```python
from build123d import *

# Parameters (mm, degrees)
F0_W     = 165
F0_H     = 100
F1_DEPTH = 2
F2_W     = 11
F2_H     = 14
F2_R     = 2
F2_R_2   = 7.5
F3_DEPTH = 25


with BuildPart() as f1:
    # F0 (on Front) → F1 (new body)
    with BuildSketch(Plane.XZ):
        Rectangle(F0_W, F0_H)
    extrude(amount=F1_DEPTH)

    # F2 (on face) → F3 (cut)
    with BuildSketch(Plane.XZ.offset(2)):
        with Locations((-5, -17)):
            Rectangle(F2_W, F2_H)
        with Locations((-3.5, 4)):
            Circle(F2_R)
        with Locations((18, -5.5)):
            Circle(F2_R_2)
        with Locations((70, -5.5)):
            Circle(F2_R_2)
    extrude(amount=-F3_DEPTH, mode=Mode.SUBTRACT)


solid = f1.part
```
The listing builds one solid part. Answer for the finished solid, in the listing's coordinates (mm). Coordinates: 2 decimals unless noted, no trailing zeros. Write each loop counter-clockwise with the first axis right and the second up, starting at its lowest first coordinate (ties: lowest second). Pieces come first, ordered by that corner, then holes. Notation, with made-up numbers: (71, -17.75) - (90, -17.75) arc R27 ccw to (90, 20.25) - close; hole circle Ø3 at (47.5, -8). An arc over 180 degrees is marked (long way). Return JSON: item names as keys, results as strings. Group by question number.
1. Determine the mould class of faces 1 (the cylindrical face through (-3.934, -1.014, 2.048)), 2 (the cylindrical face through (62.507, -1.014, -5.17)), 3 (the flat face through (-1, 0, 1)) for opening direction Z: released by +Z, released by -Z, zero draft, split by the parting line, or undercut.
2. A cutting plane is placed at B-B, the plane z = 4. Determine the outline of the cut face in (x, y).
3. Given pin 1 (12 mm diameter, centred on x = 18, z = -5.5, fed in from -Y), flat-ended and moving along its own axis, determine where the tip first touches the part or whether it passes through.
4. A cutting plane is placed at A-A, the plane x = 65.5. Determine the outline of the cut face in (y, z), plus the area to 3 significant figures.
5. Straight lines are drawn through the part: L1, parallel to Z at x = -3.5, y = -0.85; L2, parallel to Z at x = -4, y = -1; L3, parallel to X at y = -0.4, z = -17. For each, find the intervals that lie inside material, in ascending order.
6. A cutting plane is placed at C-C, the plane x = -3.5. Determine the outline of the cut face in (y, z), plus the area to 3 significant figures.
7. A cutting plane is placed at D-D, the plane y = -0.4. Determine the outline of the cut face in (x, z).
Ans:
{
 "1": {"face 1": "undercut", "face 2": "undercut", "face 3": "zero draft"},
 "2": {"outline": "(-82.5, -2) - (-5.5, -2) - (-5.5, 0) - (-82.5, 0) - close; (-1.5, -2) - (82.5, -2) - (82.5, 0) - (-1.5, 0) - close"},
 "3": {"pin 1": "through"},
 "4": {"outline": "(-2, -50) - (0, -50) - (0, -11.5) - (-2, -11.5) - close; (-2, 0.5) - (0, 0.5) - (0, 50) - (-2, 50) - close", "area": "176 mm²"},
 "5": {"L1": "-50 to -24, -10 to 2, 6 to 50", "L2": "-50 to -24, -10 to 2.06, 5.94 to 50", "L3": "-82.5 to -10.5, 0.5 to 82.5"},
 "6": {"outline": "(-2, -50) - (0, -50) - (0, -24) - (-2, -24) - close; (-2, -10) - (0, -10) - (0, 2) - (-2, 2) - close; (-2, 6) - (0, 6) - (0, 50) - (-2, 50) - close", "area": "164 mm²"},
 "7": {"outline": "(-82.5, -50) - (82.5, -50) - (82.5, 50) - (-82.5, 50) - close; hole (-10.5, -24) - (0.5, -24) - (0.5, -10) - (-10.5, -10) - close; hole circle Ø4 at (-3.5, 4); hole circle Ø15 at (18, -5.5); hole circle Ø15 at (70, -5.5)"}
}
